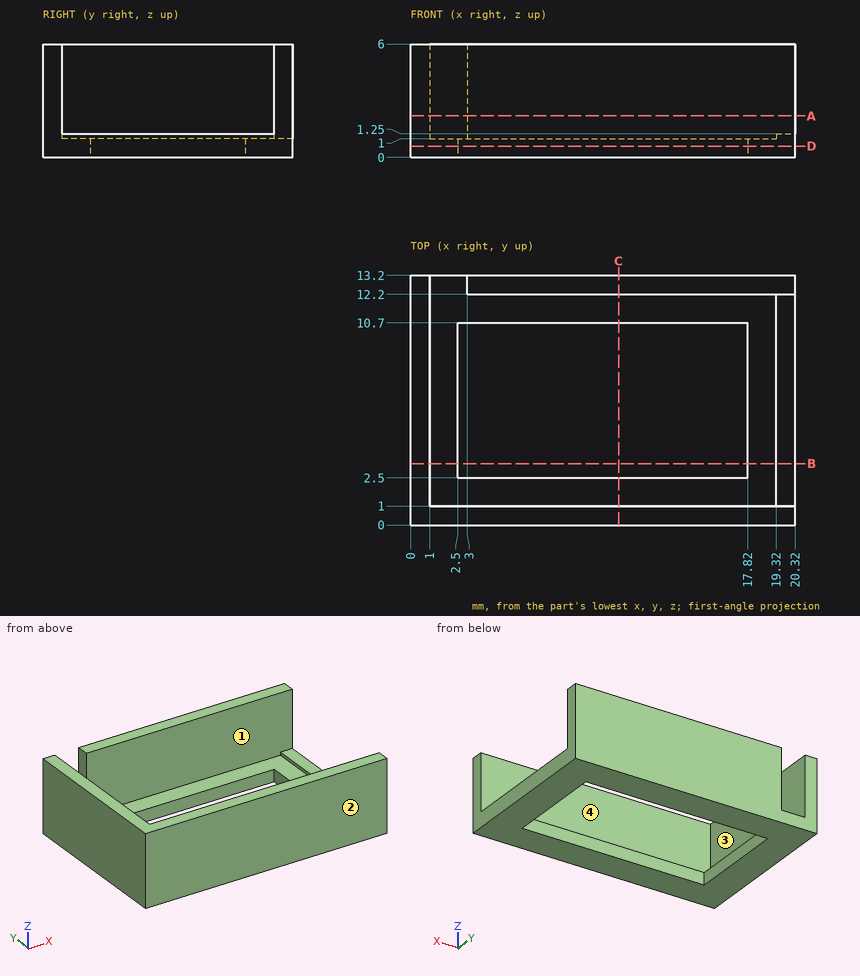
For this review, use the dimensioned drawing (mm, ordinates from the lowest corner) and the shaded views. Give positions to 0.01 mm unless a question says otherwise; leave off trailing zeros. Loops run counter-clockwise (first coordinate to the right, second up) from the corner with the lowest first, then second, coordinate; pieces in that order, holes last. Notation, with made-up numbers: (72.5, -36.5) - (129.5, -36.5) arc R5 cw to (129.5, -28.5) - close; hole circle Ø2 at (79, 83.25). An arc over 180 degrees is marked (long way). Write each question's results on one line, items separated by ' | '.
(1) For pin 1 Ø2.5 at (y, z) = (6, 3.5) entering from +X; pin 2 Ø3.5 at (x, y) = (14.5, 5.5) entering from +Z, all flat-tipped, find the tip position at first contact; note any pin that passes through.
Conclusion:
pin 1: x = 1 | pin 2: through
(2) For line 1 along Y through (x, z) = (4.25, 4.15); line 2 along Y through (x, z) = (3, 0.95); line 3 along X through (y, z) = (12.75, 5.3), list the stretches that pass through material, from the lowest coordinate up.
Conclusion:
line 1: 0 to 1, 12.2 to 13.2 | line 2: 0 to 2.5, 10.7 to 13.2 | line 3: 0 to 1, 3 to 20.32
(3) Take a section at A-A (z = 2.2). Give the boundary of the cut face in (x, y), then the cut area to 3 significant figures.
Conclusion:
outline: (0, 0) - (20.32, 0) - (20.32, 1) - (1, 1) - (1, 13.2) - (0, 13.2) - close; (3, 12.2) - (20.32, 12.2) - (20.32, 13.2) - (3, 13.2) - close | area: 49.8 mm^2
(4) Take a section at C-C (x = 11). Give the boundary of the cut face in (y, z), then the cut area to 3 significant figures.
Conclusion:
outline: (0, 0) - (2.5, 0) - (2.5, 1) - (1, 1) - (1, 6) - (0, 6) - close; (10.7, 0) - (13.2, 0) - (13.2, 6) - (12.2, 6) - (12.2, 1) - (10.7, 1) - close | area: 15.0 mm^2
(5) Take a section at B-B (y = 3.25). Give the boundary of the cut face in (x, z), then the cut area to 4 significant figures.
Conclusion:
outline: (0, 0) - (2.5, 0) - (2.5, 1) - (1, 1) - (1, 6) - (0, 6) - close; (17.82, 0) - (20.32, 0) - (20.32, 1.25) - (19.32, 1.25) - (19.32, 1) - (17.82, 1) - close | area: 10.25 mm^2
(6) Draft analysis for pull direction Y (two halves, no side actions). For the marked faces 1, 2, 3 and 4, state which applies: +Y half, -Y half, draft (parallel to the pull), parting line (faces both ways), or undercut.
Conclusion:
face 1: undercut | face 2: -Y half | face 3: draft | face 4: undercut
(7) Take a section at D-D (z = 0.6). Give the boundary of the cut face in (x, y).
Conclusion:
outline: (0, 0) - (20.32, 0) - (20.32, 13.2) - (0, 13.2) - close; hole (2.5, 2.5) - (17.82, 2.5) - (17.82, 10.7) - (2.5, 10.7) - close
